Source: three-view drawing plus pictorial views. Frame: mm from the lowest corner of the part. A direction names the side the tool comes from. Give positions to 0.01 mm unless a question says otherwise; leave off trailing zeros. Loops run counter-clockwise (first coordinate to the right, second up) from the corner with the lowest first, then second, coordinate; pieces in that order, holes last. Notation, with made-up numbers: (77.5, -14) - (111.5, -14) arc R21 ccw to (111.5, -9) - close; hole circle Ø5 at (36, 67). An arc over 180 degrees is marked (long way). Answer as a JSON object with one key per item and string values.
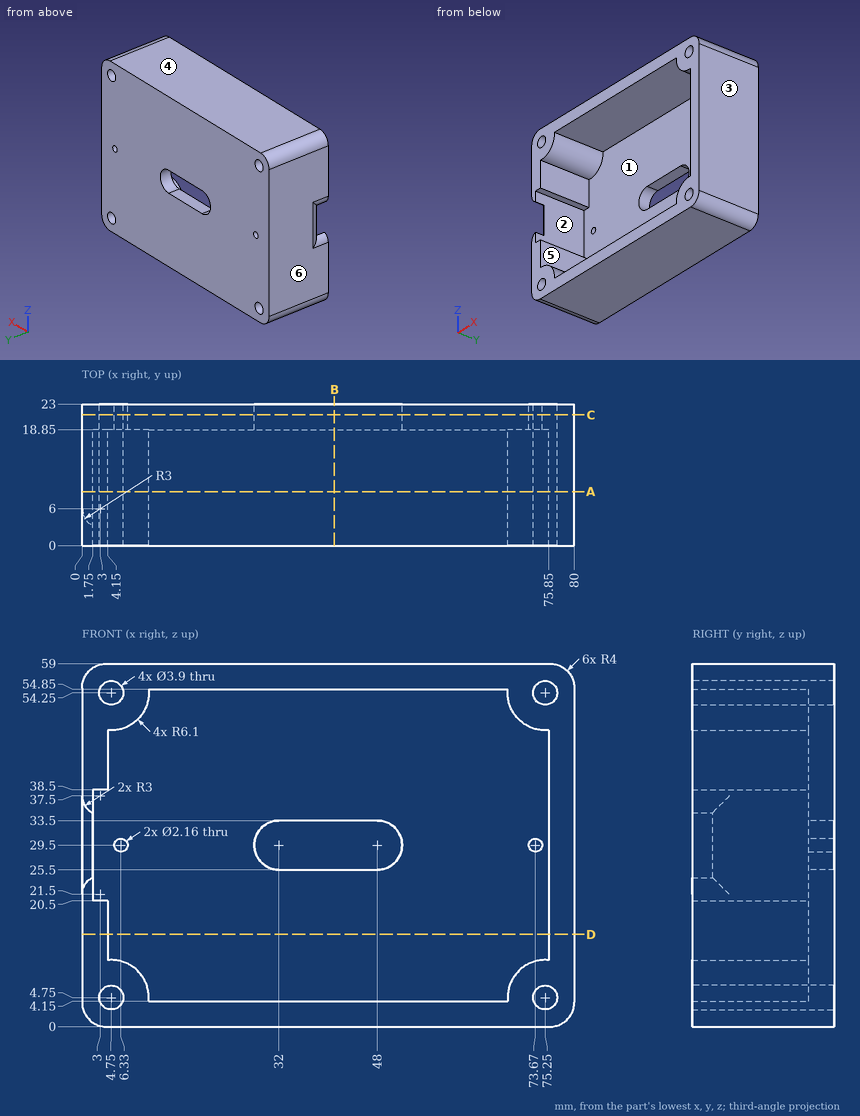
Item 1: Cut plane B-B (x = 41). Return loops of the section in (y, z), then the cut area to 3 significant figures.
Geometry check:
{"outline": "(0, 0) - (23, 0) - (23, 25.5) - (18.85, 25.5) - (18.85, 4.15) - (0, 4.15) - close; (0, 54.85) - (18.85, 54.85) - (18.85, 33.5) - (23, 33.5) - (23, 59) - (0, 59) - close", "area": "368 mm2"}
Item 2: Cut plane C-C (y = 21.25). Return loops of the section in (x, z).
Geometry check:
{"outline": "(0, 4) arc R4 ccw to (4, 0) - (76, 0) arc R4 ccw to (80, 4) - (80, 55) arc R4 ccw to (76, 59) - (4, 59) arc R4 ccw to (0, 55) - close; hole circle Ø3.9 at (4.75, 4.75); hole circle Ø3.9 at (4.75, 54.25); hole circle Ø2.16 at (6.33, 29.5); hole (32, 25.5) - (48, 25.5) arc R4 ccw to (48, 33.5) - (32, 33.5) arc R4 ccw to start; hole circle Ø2.16 at (73.67, 29.5); hole circle Ø3.9 at (75.25, 4.75); hole circle Ø3.9 at (75.25, 54.25)"}
Item 3: Mould query, pull axis Z, two halves, no side actions, for the marked faces 1, 2, 3 and 4. Classes: released by +Z, released by -Z, zero draft, split by the parting line, or undercut.
Geometry check:
{"face 1": "undercut", "face 2": "undercut", "face 3": "zero draft", "face 4": "released by +Z"}
Item 4: Material intervals for line 1 (X direction, y = 10.25, z = 54.25); line 2 (Z direction, x = 36.5, y = 8.25); line 3 (X direction, y = 4.5, z = 17), sorted ascending. Write a range as [from, to].
Geometry check:
{"line 1": "x = [0, 2.8], [6.7, 10.85], [69.15, 73.3], [77.2, 80]", "line 2": "z = [0, 4.15], [54.85, 59]", "line 3": "x = [0, 4.15], [75.85, 80]"}
Item 5: Contact query for a flat-ended pin moving along its axis: P1, Ø12, axis at x = 57, z = 42, coming from the -Y side. Output: stop coordinate, or through.
Geometry check:
{"P1": "stops at y = 18.85"}
Item 6: Access query for the marked faces 5 and 6. Directions: +Z, -Z, +X, -X, +Y, -Y. A direction counts if a zero-diameter tool reaches every point of the face in a straight line with its end or side. Return the directions, or none.
Geometry check:
{"face 5": "-Y", "face 6": "+Z, -Z, -X, +Y, -Y"}
Item 7: Cut plane D-D (z = 15). Return loops of the section in (x, y).
Geometry check:
{"outline": "(0, 0) - (4.15, 0) - (4.15, 18.85) - (75.85, 18.85) - (75.85, 0) - (80, 0) - (80, 23) - (0, 23) - close"}
Item 8: Cut plane A-A (y = 8.75). Return loops of the section in (x, z).
Geometry check:
{"outline": "(0, 4) arc R4 ccw to (4, 0) - (76, 0) arc R4 ccw to (80, 4) - (80, 55) arc R4 ccw to (76, 59) - (4, 59) arc R4 ccw to (0, 55) - close; hole (1.75, 20.5) - (4.15, 20.5) - (4.15, 10.82) arc R6.1 cw to (10.82, 4.15) - (69.18, 4.15) arc R6.1 cw to (75.85, 10.82) - (75.85, 48.18) arc R6.1 cw to (69.18, 54.85) - (10.82, 54.85) arc R6.1 cw to (4.15, 48.18) - (4.15, 38.5) - (1.75, 38.5) - close; hole circle Ø3.9 at (4.75, 4.75); hole circle Ø3.9 at (4.75, 54.25); hole circle Ø3.9 at (75.25, 4.75); hole circle Ø3.9 at (75.25, 54.25)"}
